Can you work these out from the model? Positions are in its coordinate system, mm. A direction names the side the tool comes from. Round coordinates to 2 decimals unless told otherwise and drop trailing zeros. Order: outer loops, then holes, each group sorted by start corner. A loop starts at its lowest first (then second) coordinate and runs counter-clockwise, first axis right, second up.
Q1. If we section it at D-D (y = 2): Please give me the cut outline in (x, z).
Q2. We'd pull the mould along Y, two halves only. Please class faces 3 (the face through (0, -56, 0)), 4 (the face through (11, -4.5, -10)), 5 (the face through (29, -1, 0)): pulls with the +Y half, pulls with the -Y half, needs draft (parallel to the pull), parting line crosses it, or undercut.
Q3. Will these pins go through, and if not, where does the flat tip stop? P1, Ø9, axis at x = 23, z = -7.5, coming from the +Y side; P2, Ø12, axis at x = -3, y = -17, coming from the +Z side; P3, Ø0.8, axis at x = 28.5, z = -0.5, coming from the -Y side (3 decimals); P4, Ø20.5, axis at x = 7, y = -15, coming from the +Z side.
Q4. If I drill on line 1 (X direction, y = -43, z = -11.5); line 2 (Y direction, x = -26, z = -10); line 3 (Y direction, x = 28.2, z = 0), over which ranges is the centre line in solid material (lowest first)?
Q5. If we section it at A-A (y = -43): Please give me the cut outline in (x, z), plus the area to 3 significant figures.
Q6. If we section it at B-B (x = 23): Please give me the cut outline in (y, z), plus the area to 3 significant figures.
Q7. If we section it at C-C (z = 0): Please give me the cut outline in (x, y).
Q8. For faces 1 (the face through (28.493, -35.068, 1.041)), 2 (the face through (-6.3, -12, -2.4)), which set-ups out of +Z, -Z, +X, -X, +Y, -Y let a thin tool reach every point of the face, with its end or its side?
from build123d import *

# Parameters (mm, degrees)
CYLINDER005_R           = 1.5
CYLINDER005_DEPTH       = 20
CYLINDER005_PITCH_ANGLE = 90
BOX005_W                = 10
BOX005_H                = 4
BOX005_DEPTH            = 6
CYLINDER002_R           = 8
CYLINDER002_DEPTH       = 6
CYLINDER002_PITCH_ANGLE = 90
CYLINDER001_R           = 8
CYLINDER001_DEPTH       = 6
CYLINDER001_PITCH_ANGLE = 90
CYLINDER_R              = 3.5
CYLINDER_DEPTH          = 50
CYLINDER_ROLL_ANGLE     = 90
CYLINDER006_R           = 1.5
CYLINDER006_DEPTH       = 20
CYLINDER006_PITCH_ANGLE = 90
BOX003_W                = 35.5
BOX003_H                = 1
BOX003_DEPTH            = 5
BOX004_W                = 35.5
BOX004_H                = 1
BOX004_DEPTH            = 5
BOX006_W                = 22
BOX006_H                = 1
BOX006_DEPTH            = 10
BOX002_W                = 1
BOX002_H                = 112
BOX002_DEPTH            = 10
BOX_W                   = 56
BOX_H                   = 110
BOX_DEPTH               = 25
BOX001_W                = 58
BOX001_H                = 112
BOX001_DEPTH            = 25
CHAMFER_SIZE            = 1
FILLET_R                = 1


with BuildPart() as cylinder005:
    # Cylinder005 → Cylinder005 (new body)
    with BuildSketch(Plane.XY):
        Circle(CYLINDER005_R)
    extrude(amount=CYLINDER005_DEPTH)


with BuildPart() as cylinder005_1:
    # Cylinder005 pitch: moved
    add(cylinder005.part.rotate(Axis((0, 0, 0), (0, 1, 0)), CYLINDER005_PITCH_ANGLE))


with BuildPart() as cylinder005_2:
    # Cylinder005 placement: moved
    add(cylinder005_1.part.moved(Location((19.5, -28, -7.5))))


with BuildPart() as obj1:
    # Box005 → Box005 (new body)
    with BuildSketch(Plane(origin=(24, -30, -3), x_dir=(1, 0, 0), z_dir=(0, 0, 1))):
        with Locations((5, 2)):
            Rectangle(BOX005_W, BOX005_H)
    extrude(amount=BOX005_DEPTH)


with BuildPart() as obj2:
    # Cylinder002 → Cylinder002 (new body)
    with BuildSketch(Plane.XY):
        Circle(CYLINDER002_R)
    extrude(amount=CYLINDER002_DEPTH)


with BuildPart() as obj2_1:
    # Cylinder002 pitch: moved
    add(obj2.part.rotate(Axis((0, 0, 0), (0, 1, 0)), CYLINDER002_PITCH_ANGLE))


with BuildPart() as obj2_2:
    # Cylinder002 placement: moved
    add(obj2_1.part.moved(Location((25.5, -43, 0))))


with BuildPart() as obj3:
    # Cylinder001 → Cylinder001 (new body)
    with BuildSketch(Plane.XY):
        Circle(CYLINDER001_R)
    extrude(amount=CYLINDER001_DEPTH)


with BuildPart() as obj3_1:
    # Cylinder001 pitch: moved
    add(obj3.part.rotate(Axis((0, 0, 0), (0, 1, 0)), CYLINDER001_PITCH_ANGLE))


with BuildPart() as obj3_2:
    # Cylinder001 placement: moved
    add(obj3_1.part.moved(Location((25.5, -12.7, 0))))


with BuildPart() as antenna_hole:
    # Cylinder → Cylinder (new body)
    with BuildSketch(Plane.XY):
        Circle(CYLINDER_R)
    extrude(amount=CYLINDER_DEPTH)


with BuildPart() as antenna_hole_1:
    # Cylinder roll: moved
    add(antenna_hole.part.rotate(Axis((0, 0, 0), (1, 0, 0)), CYLINDER_ROLL_ANGLE))


with BuildPart() as antenna_hole_2:
    # Cylinder placement: moved
    add(antenna_hole_1.part.moved(Location((23, 86.9, -7.5))))


with BuildPart() as obj4:
    # Cylinder006 → Cylinder006 (new body)
    with BuildSketch(Plane.XY):
        Circle(CYLINDER006_R)
    extrude(amount=CYLINDER006_DEPTH)


with BuildPart() as obj4_1:
    # Cylinder006 pitch: moved
    add(obj4.part.rotate(Axis((0, 0, 0), (0, 1, 0)), CYLINDER006_PITCH_ANGLE))


with BuildPart() as obj4_2:
    # Cylinder006 placement: moved
    add(obj4_1.part.moved(Location((19.5, -28, 7.5))))

    # Fusion001: union Cylinder005, obj1, obj2, obj3, antenna_hole
    add(cylinder005_2.part)
    add(obj1.part)
    add(obj2_2.part)
    add(obj3_2.part)
    add(antenna_hole_2.part)


with BuildPart() as obj5:
    # Box003 → Box003 (new body)
    with BuildSketch(Plane(origin=(-6.7, -4.5, -12.4), x_dir=(1, 0, 0), z_dir=(0, 0, 1))):
        with Locations((17.75, 0.5)):
            Rectangle(BOX003_W, BOX003_H)
    extrude(amount=BOX003_DEPTH)


with BuildPart() as obj6:
    # Box004 → Box004 (new body)
    with BuildSketch(Plane(origin=(-6.7, -24, -12.4), x_dir=(1, 0, 0), z_dir=(0, 0, 1))):
        with Locations((17.75, 0.5)):
            Rectangle(BOX004_W, BOX004_H)
    extrude(amount=BOX004_DEPTH)


with BuildPart() as obj7:
    # Box006 → Box006 (new body)
    with BuildSketch(Plane(origin=(-28, -25, -12.4), x_dir=(1, 0, 0), z_dir=(0, 0, 1))):
        with Locations((11, 0.5)):
            Rectangle(BOX006_W, BOX006_H)
    extrude(amount=BOX006_DEPTH)


with BuildPart() as obj8:
    # Box002 → Box002 (new body)
    with BuildSketch(Plane(origin=(-7, -56, -12.4), x_dir=(1, 0, 0), z_dir=(0, 0, 1))):
        with Locations((0.5, 56)):
            Rectangle(BOX002_W, BOX002_H)
    extrude(amount=BOX002_DEPTH)

    # Fusion: union obj5, obj6, obj7
    add(obj5.part)
    add(obj6.part)
    add(obj7.part)


with BuildPart() as cubo_interior:
    # Box → Box (new body)
    with BuildSketch(Plane(origin=(-28, -55, -11.9), x_dir=(1, 0, 0), z_dir=(0, 0, 1))):
        with Locations((28, 55)):
            Rectangle(BOX_W, BOX_H)
    extrude(amount=BOX_DEPTH)


with BuildPart() as obj9:
    # Box001 → Box001 (new body)
    with BuildSketch(Plane(origin=(-29, -56, -12.5), x_dir=(1, 0, 0), z_dir=(0, 0, 1))):
        with Locations((29, 56)):
            Rectangle(BOX001_W, BOX001_H)
    extrude(amount=BOX001_DEPTH)

    # Cut: cut Cubo_interior
    add(cubo_interior.part, mode=Mode.SUBTRACT)

    # Fusion002: union obj8
    add(obj8.part)

    # Cut001: cut obj4
    add(obj4_2.part, mode=Mode.SUBTRACT)

    # Chamfer
    chamfer_edges = [obj9.edges().sort_by_distance(p)[0] for p in [
        (-7, -55, -7.15),
        (-6, -55, -7.15),
        (28, -24, -9.65),
        (28, -23, -9.65),
        (28, -3.5, -9.65),
        (28, -4.5, -9.65),
        (-6, 55, -7.15),
        (-7, 55, -7.15),
        (-28, -24, -7.15),
        (-28, -25, -7.15),
        (-7, -25, -7.15),
        (-6, -3.5, -9.65),
        (-6, -4.5, -9.65),
        (-6, -23, -9.65),
        (-6, -24, -9.65),
        (-7, -24, -7.15),
    ]]
    chamfer(chamfer_edges, length=CHAMFER_SIZE)

    # Fillet
    fillet_edges = [obj9.edges().sort_by_distance(p)[0] for p in [
        (-29, -56, 0),
        (-29, 56, 0),
        (29, 56, 0),
        (29, -56, 0),
    ]]
    fillet(fillet_edges, radius=FILLET_R)


solid = obj9.part
Solution:
1. outline: (-29, -12.5) - (29, -12.5) - (29, 12.5) - (28, 12.5) - (28, -11.9) - (-6, -11.9) - (-6, -2.4) - (-7, -2.4) - (-7, -11.9) - (-28, -11.9) - (-28, 12.5) - (-29, 12.5) - close
2. face 3: pulls with the -Y half
2. face 4: undercut
2. face 5: needs draft
3. P1: stops at y = 56
3. P2: stops at z = -2.4
3. P3: stops at y = -55.995
3. P4: stops at z = -7.4
4. line 1: x = -29 to -28, -7 to -6, 28 to 29
4. line 2: y = -56 to -55, -25 to -24, 55 to 56
4. line 3: y = -55.98 to -51, -35 to -30, -26 to -20.7, -4.7 to 55.98
5. outline: (-29, -12.5) - (29, -12.5) - (29, -8) - (28, -8) - (28, -11.9) - (-6, -11.9) - (-6, -2.4) - (-7, -2.4) - (-7, -11.9) - (-28, -11.9) - (-28, 12.5) - (-29, 12.5) - close; (28, 8) - (29, 8) - (29, 12.5) - (28, 12.5) - close
5. area: 77.1 mm2
6. outline: (-56, -12.5) - (56, -12.5) - (56, -11) - (55, -11) - (55, -11.9) - (-3.5, -11.9) - (-3.5, -7.4) - (-4.5, -7.4) - (-4.5, -11.9) - (-23, -11.9) - (-23, -7.4) - (-24, -7.4) - (-24, -11.9) - (-55, -11.9) - (-55, 12.5) - (-56, 12.5) - close; (55, -4) - (56, -4) - (56, 12.5) - (55, 12.5) - close
6. area: 118 mm2
7. outline: (-29, -55) arc R1 ccw to (-28, -56) - (28, -56) arc R1 ccw to (29, -55) - (29, -51) - (28, -51) - (28, -55) - (-28, -55) - (-28, 55) - (28, 55) - (28, -4.7) - (29, -4.7) - (29, 55) arc R1 ccw to (28, 56) - (-28, 56) arc R1 ccw to (-29, 55) - close; (28, -35) - (29, -35) - (29, -30) - (28, -30) - close; (28, -26) - (29, -26) - (29, -20.7) - (28, -20.7) - close
8. face 1: +X
8. face 2: +Z
